from build123d import *

# Parameters (mm, degrees)
SKETCH1_R           = 3
BOSS_EXTRUDE1_DEPTH = 22
BOSS_EXTRUDE2_DEPTH = 12
CHAMFER1_SIZE       = 0.15


with BuildPart() as part:
    # Sketch1 → Boss-Extrude1 (new body)
    with BuildSketch(Plane.XY):
        Circle(SKETCH1_R)
    extrude(amount=BOSS_EXTRUDE1_DEPTH)

    # Sketch2 → Boss-Extrude2 (add)
    with BuildSketch(Plane.XY.offset(22)):
        with BuildLine():
            ThreePointArc((1.658312395, -2.5), (0, 3), (-1.658312395, -2.5))
            Line((-1.658312395, -2.5), (1.658312395, -2.5))
        make_face()
    extrude(amount=BOSS_EXTRUDE2_DEPTH)

    # Chamfer1
    chamfer1_edges = [part.edges().sort_by_distance(p)[0] for p in [
        (0, 3, 34),
    ]]
    chamfer(chamfer1_edges, length=CHAMFER1_SIZE)


solid = part.part
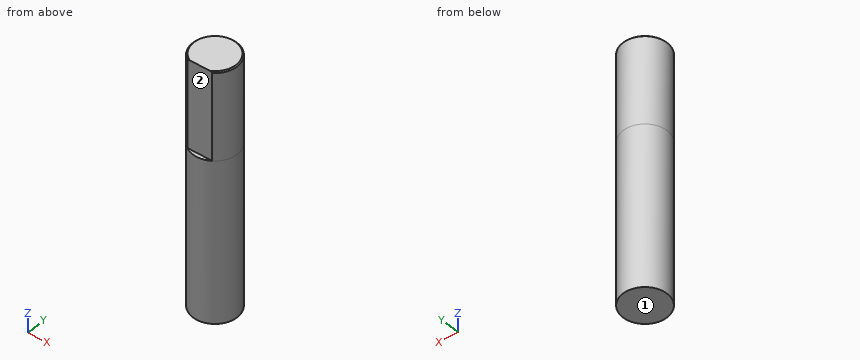
Source: CAD feature listing. Evaluate the final solid. Frame: model axes, mm. Face numbers are marked on the shaded views. A direction names the side the tool comes from. Round coordinates to 2 decimals unless told otherwise and drop trailing zeros. Write each loop counter-clockwise with the first axis right and the second up, starting at its lowest first coordinate (ties: lowest second). Pieces come first, ordered by that corner, then holes. Notation, with made-up numbers: M -18,81.25 L 4,81.25 A16 cw 4,91.25 Z; hole C 7.5,-37.75 d8. An arc over 180 degrees is marked long. One line per item, written item: value. Start each with the question number.
Item 1: Section query A-A (x = 0). Return the cut outline in (y, z).
Item 2: Set-up query: the marked faces 1 and 2. Return all of +Z, -Z, +X, -X, +Y, -Y with unobstructed straight access to the full face (end or side cutting, diameter ignored); none if empty.
Item 3: Pin query (flat end, axial travel): pin 1 (1 mm diameter, centred on x = -2, z = 8, fed in from -Y); pin 2 (1 mm diameter, centred on x = -1, z = 13.5, fed in from +Y); pin 3 (1.7 mm diameter, centred on x = 1, z = 28, fed in from -Y). Return the tip coordinate at first contact, or that it passes through.
Item 4: Section query B-B (z = 9.5). Return the cut outline in (x, y), plus the area to 3 significant figures.
Item 5: Ray query, L1, parallel to Y at x = -0.05, z = 29; L2, parallel to Y at x = 2.5, z = 5. Return the intervals inside material, ascending. Write a range as from..to.
Result set:
1. outline: M -3,0 L 3,0 L 3,33.85 L 2.85,34 L -2.5,34 L -2.5,22 L -3,22 Z
2. face 1: -Z, +X, -X, +Y, -Y
2. face 2: +Z, +X, -X, -Y
3. pin 1: stops at y = -2.6
3. pin 2: stops at y = 2.96
3. pin 3: stops at y = -2.5
4. outline: C 0,0 d6
4. area: 28.3 mm²
5. L1: y = -2.5..3
5. L2: y = -1.66..1.66
